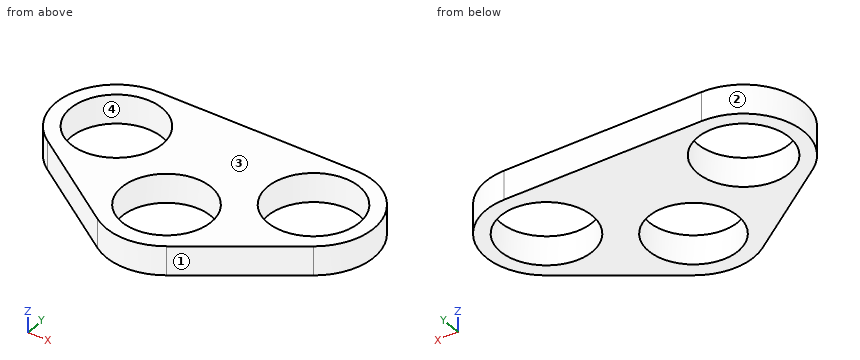
from build123d import *

# Parameters (mm, degrees)
CROQUIS1_R              = 12.5
CROQUIS1_R_2            = 9.247768435
CROQUIS1_R_3            = 9.5
SALIENTE_EXTRUIR1_DEPTH = 6


with BuildPart() as part:
    # Croquis1 → Saliente-Extruir1 (new body)
    # profile 1 of 6: a face of its own
    with BuildSketch(Plane.XY):
        with BuildLine():
            Line((20.478801107, 26.839410909), (-20.478801107, 26.839410909))
            ThreePointArc((-20.478801107, 26.839410909), (-11.639966342, 23.178245674), (-7.978801107, 14.339410909))
            ThreePointArc((-7.978801107, 14.339410909), (-8.557339261, 10.580588295), (-10.239400698, 7.169705249))
            ThreePointArc((-10.239400698, 7.169705249), (-6.8e-08, 12.5), (10.239400619, 7.169705361))
            ThreePointArc((10.239400619, 7.169705361), (9.391165666, 20.111268523), (20.478801107, 26.839410909))
        make_face()
    # profile 2 of 6: a face of its own
    with BuildSketch(Plane.XY):
        with BuildLine():
            ThreePointArc((-10.239400698, 7.169705249), (-18.30819901, 2.029313974), (-27.648506562, 4.100010355))
            Line((-27.648506562, 4.100010355), (-7.169705454, -10.239400554))
            ThreePointArc((-7.169705454, -10.239400554), (-12.310096891, -2.170602344), (-10.239400698, 7.169705249))
        make_face()
    # profile 3 of 6: a face of its own
    with BuildSketch(Plane.XY):
        with BuildLine():
            ThreePointArc((27.648506562, 4.100010355), (18.308198943, 2.029313986), (10.239400619, 7.169705361))
            ThreePointArc((10.239400619, 7.169705361), (11.921461902, 3.758822439), (12.5, 0))
            ThreePointArc((12.5, 0), (11.087635415, -5.771857665), (7.169705454, -10.239400554))
            Line((7.169705454, -10.239400554), (27.648506562, 4.100010355))
        make_face()
    # profile 4 of 6: a face of its own
    with BuildSketch(Plane.XY):
        Circle(CROQUIS1_R)
        Circle(CROQUIS1_R_2, mode=Mode.SUBTRACT)
    # profile 5 of 6: a face of its own
    with BuildSketch(Plane.XY):
        with Locations((-20.478801107, 14.339410909)):
            Circle(CROQUIS1_R)
        with Locations((-20.478801107, 14.339410909)):
            Circle(CROQUIS1_R_3, mode=Mode.SUBTRACT)
    # profile 6 of 6: a face of its own
    with BuildSketch(Plane.XY):
        with Locations((20.478801107, 14.339410909)):
            Circle(CROQUIS1_R)
        with Locations((20.478801107, 14.339410909)):
            Circle(CROQUIS1_R_3, mode=Mode.SUBTRACT)
    extrude(amount=SALIENTE_EXTRUIR1_DEPTH)


solid = part.part
Work out the finished part from the listing and answer in its coordinate system (mm). Face numbers are marked on the shaded views. Round coordinates to 2 decimals unless told otherwise and drop trailing zeros. Write each loop counter-clockwise with the first axis right and the second up, starting at its lowest first coordinate (ties: lowest second). Pieces come first, ordered by that corner, then holes.
1) A cutting plane is placed at C-C (z = 3.5). Give the vertices of the cut face in (x, y), plus the area to 3 significant figures.
2) Given pin 1 Ø15 at (x, y) = (20.48, 14.34) entering from +Z; pin 2 Ø3 at (y, z) = (-6.5, 3.5) entering from -X; pin 3 Ø2 at (x, z) = (-24.5, 4.5) entering from -Y, each flat-ended and moving along its own axis, determine where each tip first touches the part or whether it passes through.
3) A cutting plane is placed at B-B (y = -7.5). Give the vertices of the cut face in (x, z).
4) A cutting plane is placed at A-A (x = 0). Give the vertices of the cut face in (y, z), plus the area to 3 significant figures.
5) The mould has two halves that part along X. Classify the marked faces 1, 2, 3 and 4: pulls with the +X half, pulls with the -X half, needs draft (parallel to the pull), parting line crosses it, or undercut.
6) Straight lines are drawn through the part: line 1 (X direction, y = 14.5, z = 1.4); line 2 (X direction, y = 8, z = 1.5); line 3 (Y direction, x = 0, z = 3.75). For each, find the intervals that lie inside material, in ascending order.
7) A cutting plane is placed at D-D (y = 22.5). Give the vertices of the cut face in (x, z).
Completed:
1. outline: (-27.65, 4.1) - (-7.17, -10.24) arc R12.5 ccw to (7.17, -10.24) - (27.65, 4.1) arc R12.5 ccw to (20.48, 26.84) - (-20.48, 26.84) arc R12.5 ccw to start; hole circle Ø19 at (-20.48, 14.34); hole circle Ø18.5 at (0, 0); hole circle Ø19 at (20.48, 14.34)
1. area: 1,090 mm2
2. pin 1: passes through
2. pin 2: stops at x = -14.65
2. pin 3: stops at y = 1.2
3. outline: (-11.08, 0) - (-5.41, 0) - (-5.41, 6) - (-11.08, 6) - close; (5.41, 0) - (11.08, 0) - (11.08, 6) - (5.41, 6) - close
4. outline: (-12.5, 0) - (-9.25, 0) - (-9.25, 6) - (-12.5, 6) - close; (9.25, 0) - (26.84, 0) - (26.84, 6) - (9.25, 6) - close
4. area: 125 mm2
5. face 1: pulls with the +X half
5. face 2: pulls with the -X half
5. face 3: needs draft
5. face 4: undercut
6. line 1: x = -32.98 to -29.98, -10.98 to 10.98, 29.98 to 32.98
6. line 2: x = -31.25 to -27.55, -13.4 to -4.64, 4.64 to 13.4, 27.55 to 31.25
6. line 3: y = -12.5 to -9.25, 9.25 to 26.84
7. outline: (-29.95, 0) - (-25.34, 0) - (-25.34, 6) - (-29.95, 6) - close; (-15.62, 0) - (15.62, 0) - (15.62, 6) - (-15.62, 6) - close; (25.34, 0) - (29.95, 0) - (29.95, 6) - (25.34, 6) - close
